```python
from build123d import *

# Parameters (mm, degrees)
F0_R        = 8.4292164968
F1_DEPTH    = 63.5
F0_W        = 25.4
F0_H        = 19.05
F2_DEPTH    = 25.4
F0_H_2      = 4.7498
F0_H_3      = 4.7752
F4_DEPTH    = 25.4
F5_DEPTH    = 25.4
F6_T1_DEPTH = 88.9
F6_T4_ANGLE = 180
F7_T        = 2.54
F7_T3_DEPTH = 24.13
F7_T5_DEPTH = 55.88
F7_T7_DEPTH = 55.7790871697
F7_T9_DEPTH = 34.6589952471


# Not quite as in the source:
# - a fillet or chamfer that OpenCascade refuses, or shapes differently, is made with other operations: its cross-section is extruded or revolved along the edge and cut away or added
# - a feature of the source that left no trace in its solid (it failed there, or was rolled back) is left out
# - a shell that OpenCascade refuses in one call is made with other operations: the cavity is built on its own and cut out


with BuildPart() as f1:
    # F0 (on Front) → F1 (new body, symmetric)
    with BuildSketch(Plane.XZ):
        Polygon((-41.275, -9.525), (41.275, -9.525), (41.275, 9.525), (22.225, 9.525), (-41.275, 9.525), align=None)
        with Locations((-17.5714660436, 0)):
            Circle(F0_R, mode=Mode.SUBTRACT)
    extrude(amount=F1_DEPTH, both=True)

    # F0 (on Front) → F2 (join, symmetric)
    with BuildSketch(Plane.XZ):
        with BuildLine():
            Line((60.325, 61.9252), (57.15, 61.9252))
            ThreePointArc((57.15, 61.9252), (32.4542956671, 51.6959043329), (22.225, 27.0002))
            Line((22.225, 27.0002), (22.225, 9.525))
            Line((22.225, 9.525), (41.275, 9.525))
            Line((41.275, 9.525), (41.275, 27.0002))
            ThreePointArc((41.275, 27.0002), (45.9246798487, 38.2255201513), (57.15, 42.8752))
            Line((57.15, 42.8752), (60.325, 42.8752))
            Line((60.325, 42.8752), (60.325, 61.9252))
        make_face()
        with Locations((73.025, 52.4002)):
            Rectangle(F0_W, F0_H)
    extrude(amount=F2_DEPTH, both=True)

    # F0 (on Front) → F3 (revolve)
    with BuildSketch(Plane.XZ):
        Polygon((85.725, 66.675), (85.725, 61.9252), (85.725, 42.8752), (85.725, 38.1), (111.125, 38.1), (111.125, 66.675), align=None)
    revolve(axis=Axis((85.725, 0, 52.3875), (0, 0, 1)))

    # F0 (on Front) → F4 (join)
    with BuildSketch(Plane.XZ):
        with Locations((73.025, 64.3001)):
            Rectangle(F0_W, F0_H_2)
        with Locations((73.025, 40.4876)):
            Rectangle(F0_W, F0_H_3)
    extrude(amount=F4_DEPTH)

    # F0 (on Front) → F5 (join)
    with BuildSketch(Plane.XZ):
        with Locations((73.025, 40.4876)):
            Rectangle(F0_W, F0_H_3)
        with Locations((73.025, 64.3001)):
            Rectangle(F0_W, F0_H_2)
    extrude(amount=-F5_DEPTH)

    # F6: fillet of radius 25.4 on 3 edges, made by hand

    # F6_s2 → F6_t1 (cut)
    with BuildSketch(Plane.YZ.offset(-3.175)):
        with BuildLine():
            ThreePointArc((-25.4, 41.275), (-17.9605122421, 59.2355122421), (0, 66.675))
            Line((0, 66.675), (-25.4, 66.675))
            Line((-25.4, 66.675), (-25.4, 41.275))
        make_face()
        with BuildLine():
            ThreePointArc((0, 66.675), (17.9605122421, 59.2355122421), (25.4, 41.275))
            Line((25.4, 41.275), (25.4, 66.675))
            Line((25.4, 66.675), (0, 66.675))
        make_face()
    extrude(amount=F6_T1_DEPTH, mode=Mode.SUBTRACT)

    # F6_s3 → F6_t4 (revolve, cut)
    with BuildSketch(Plane.YZ.offset(85.725)):
        with BuildLine():
            ThreePointArc((0, 66.675), (17.9605122421, 59.2355122421), (25.4, 41.275))
            Line((25.4, 41.275), (25.4, 66.675))
            Line((25.4, 66.675), (0, 66.675))
        make_face()
    revolve(axis=Axis((85.725, 0, 66.675), (0, 0, -1)), revolution_arc=F6_T4_ANGLE, mode=Mode.SUBTRACT)

    # F7: shell of thickness 2.54, made by hand


with BuildPart() as f7_core1:
    # F7_t2: copy of F1
    add(f1.part)

    # the walls: a layer under each face that stays
    f7_faces = [f7_core1.faces().sort_by_distance(p)[0] for p in [
        (0, 0, -9.525),
        (0, 63.5, 0),
        (41.275, 0, 8.7376),
        (0, -63.5, 0),
        (-41.275, 0, 0),
        (0, 0, 9.525),
        (-26.0006825404, 0, 0),
        (36.214543408, 25.4, 25.4),
        (45.9246798487, 0, 38.2255201513),
        (36.214543408, -25.4, 25.4),
        (22.225, 0, 18.2626),
        (55.5002346295, 17.9605122421, 59.2355122421),
        (32.4542956671, 0, 51.6959043329),
        (55.5002346295, -17.9605122421, 59.2355122421),
        (58.7375, 0, 42.8752),
        (60.325, 0, 64.3001),
        (58.7375, 0, 61.9252),
        (60.325, 0, 40.4876),
        (73.025, 25.4, 39.6875),
        (103.6855122422, -1e-10, 59.2355122421),
        (73.025, -25.4, 39.6875),
        (111.125, 0, 39.6875),
    ]]
    thicken(f7_faces, amount=-F7_T, mode=Mode.SUBTRACT)

    # F7_s4 → F7_t3 (cut)
    with BuildSketch(Plane.YZ.offset(19.685)):
        Polygon((25.4254, 9.5504), (25.4, 6.985), (22.86, 6.985), (22.86, 9.525), align=None)
        Polygon((-25.4254, 9.5504), (-25.4, 6.985), (-22.86, 6.985), (-22.86, 9.525), align=None)
    extrude(amount=F7_T3_DEPTH, mode=Mode.SUBTRACT)

    # F7_s6 → F7_t5 (cut)
    with BuildSketch(Plane.XZ.offset(-27.94)):
        Polygon((22.1996, 9.5504), (22.225, 6.985), (24.765, 6.985), (24.765, 9.525), align=None)
    extrude(amount=F7_T5_DEPTH, mode=Mode.SUBTRACT)

    # F7_s8 → F7_t7 (cut)
    with BuildSketch(Plane.XZ.offset(-27.8895435848)):
        Polygon((60.2996, 42.8498), (60.325, 45.4152), (62.865, 45.4152), (62.865, 42.8752), align=None)
    extrude(amount=F7_T7_DEPTH, mode=Mode.SUBTRACT)

    # F7_s10 → F7_t9 (cut)
    with BuildSketch(Plane.XZ.offset(-17.3294976236)):
        Polygon((60.2996, 61.9506), (62.865, 61.9252), (62.865, 59.3852), (60.325, 59.3852), align=None)
    extrude(amount=F7_T9_DEPTH, mode=Mode.SUBTRACT)


with BuildPart() as f1_1:
    add(f1.part)

    # what is left inside the walls is the cavity
    f7_cavity = [f7_core1.part.solids().sort_by_distance(p)[0] for p in [
        (-28.566083, -20.32, 0),
        (14.810641, 20.32, -6.9596),
    ]]
    add(f7_cavity, mode=Mode.SUBTRACT)


solid = f1_1.part
```
Could you check a few things on this model? Use its own coordinates, in mm. A direction names the side the tool comes from. Give positions to 0.01 mm unless a question says otherwise; leave off trailing zeros. Write each loop counter-clockwise with the first axis right and the second up, starting at its lowest first coordinate (ties: lowest second). Pieces come first, ordered by that corner, then holes. Notation, with made-up numbers: (43, 11) -> (55, 11) arc R27 cw to (55, 44) -> close; hole circle Ø2 at (16, 51). An arc over 180 degrees is marked (long way). Write each question's results on one line, items separated by ' | '.
1. I want a section at D-D, the plane x = 75. Write out the boundary of the cut face in (y, z) (3 decimals), then the cut area to 3 significant figures.
Check sheet entries:
outline: (-25.4, 38.1) -> (-22.86, 38.1) -> (-22.86, 41.275) arc R22.86 cw to (22.86, 41.275) -> (22.86, 38.1) -> (25.4, 38.1) -> (25.4, 41.275) arc R25.4 ccw to (-25.4, 41.275) -> close | area: 209 mm²
2. Will these pins go through, and if not, where does the flat tip stop? pin 1 Ø16.5 at (x, z) = (33, 20.5) entering from +Y; pin 2 Ø6 at (x, y) = (73, 6) entering from -Z; pin 3 Ø6.5 at (x, y) = (59, -3.5) entering from +Z.
Check sheet entries:
pin 1: stops at y = 25.4 | pin 2: stops at z = 62.29 | pin 3: stops at z = 66.67
3. I want a section at C-C, the plane y = 55.5. Write out the boundary of the cut face in (x, z) (3 decimals), then the cut area to 3 significant figures.
Check sheet entries:
outline: (-41.275, -9.525) -> (41.275, -9.525) -> (41.275, 9.525) -> (-41.275, 9.525) -> close; hole (-38.735, -6.985) -> (-26.029, -6.985) arc R10.969 cw to (-26.029, 6.985) -> (-38.735, 6.985) -> close; hole circle Ø16.858 at (-17.571, 0); hole (-9.114, -6.985) -> (38.735, -6.985) -> (38.735, 6.985) -> (-9.114, 6.985) arc R10.969 cw to start | area: 551 mm²
4. I need wall thicknesses on L1, parallel to Z at x = -30, y = 14.5 (3 decimals); L2, parallel to X at y = -17, z = 13.5 (3 decimals); L3, parallel to Y at x = 32, z = -2. Which ranges of each line are inside material? Lowest first, please.
Check sheet entries:
L1: z = -9.525 to -6.985, 6.985 to 9.525 | L2: x = 22.225 to 24.765, 38.735 to 41.275 | L3: y = -63.5 to -60.96, 60.96 to 63.5
5. I want a section at B-B, the plane z = 0. Write out the boundary of the cut face in (x, y) (3 decimals), then the cut area to 3 significant figures.
Check sheet entries:
outline: (-41.275, -63.5) -> (-26.001, -63.5) -> (-26.001, 63.5) -> (-41.275, 63.5) -> close; (-9.142, -63.5) -> (41.275, -63.5) -> (41.275, 63.5) -> (-9.142, 63.5) -> close; hole (-38.735, -60.96) -> (-28.541, -60.96) -> (-28.541, 60.96) -> (-38.735, 60.96) -> close; hole (-6.602, -60.96) -> (38.735, -60.96) -> (38.735, 60.96) -> (-6.602, 60.96) -> close | area: 1,570 mm²
6. I want a section at A-A, the plane x = 3. Write out the boundary of the cut face in (y, z) (3 decimals).
Check sheet entries:
outline: (-63.5, -9.525) -> (63.5, -9.525) -> (63.5, 9.525) -> (-63.5, 9.525) -> close; hole (-60.96, -6.985) -> (60.96, -6.985) -> (60.96, 6.985) -> (-60.96, 6.985) -> close
7. On a 3-axis mill with a long thin cutter (end or side, diameter ignored), from which of +Z, -Z, +X, -X, +Y, -Y can I reach the whole of each face in a straight line? I mean faces 1 (the flat face through (60.325, 0, 64)), 2 (the flat face through (89, -23, 38.1)), 3 (the flat face through (-32, -1, -6.985)), 4 (the flat face through (62.865, 0, 61)). Say none if no direction works.
Check sheet entries:
face 1: +Z, -X, +Y, -Y | face 2: -Z, +X, +Y, -Y | face 3: none | face 4: -Z
8. If we mould it in two halves opening along Y, with no side actions, what happens to faces 5 (the flat face through (-1, -63.5, 0)), 6 (the flat face through (60, 0, 45.415)), 7 (the flat face through (1, -1, 9.525)), 8 (the cylindrical face through (111.12, -0.56, 39.71))? For each: released by +Y, released by -Y, zero draft, split by the parting line, or undercut.
Check sheet entries:
face 5: released by -Y | face 6: undercut | face 7: zero draft | face 8: split by the parting line
